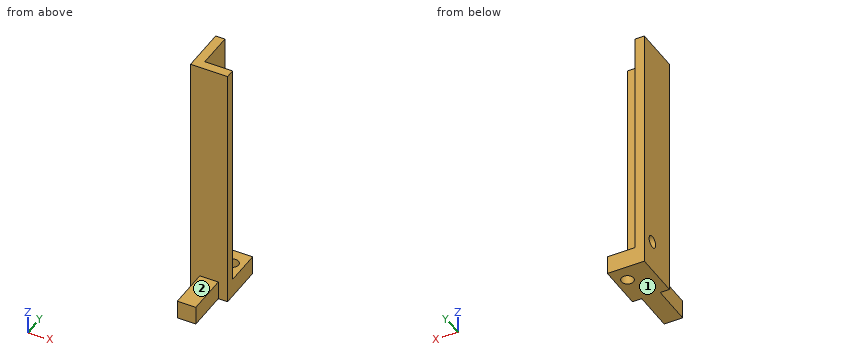
```python
from build123d import *

# Parameters (mm, degrees)
BOSS_EXTRUDE1_DEPTH      = 10
SKETCH2_W                = 30
SKETCH2_H                = 25
BOSS_EXTRUDE2_DEPTH      = 5
BOSS_EXTRUDE3_DEPTH      = 5
BOSS_EXTRUDE4_DEPTH      = 105
SKETCH7_R                = 3.25
CUT_EXTRUDE10_DEPTH      = 15
CUT_EXTRUDE10_DEPTH_BACK = 13
SKETCH8_R                = 3.25
CUT_EXTRUDE11_DEPTH      = 17
CUT_EXTRUDE11_DEPTH_BACK = 14


with BuildPart() as part:
    # Sketch1 → Boss-Extrude1 (new body)
    with BuildSketch(Plane(origin=(0, 0, 0), x_dir=(0, 0, -1), z_dir=(1, 0, 0))):
        Polygon((0, 0), (-10, 0), (-10, -20), (-30, -20), (-30, -25), (-10, -25), (-10, -47.38), (0, -47.38), align=None)
    extrude(amount=BOSS_EXTRUDE1_DEPTH)

    # Sketch2 → Boss-Extrude2 (add)
    with BuildSketch(Plane.ZY):
        with Locations((15, -12.5)):
            Rectangle(SKETCH2_W, SKETCH2_H)
    extrude(amount=BOSS_EXTRUDE2_DEPTH)

    # Sketch3 → Boss-Extrude3 (add)
    with BuildSketch(Plane(origin=(10, 0, 0), x_dir=(0, 0, -1), z_dir=(1, 0, 0))):
        Polygon((-10, 0), (-10, -20), (-30, -20), (-30, -25), (-10, -25), (0, -25), (0, 0), align=None)
    extrude(amount=BOSS_EXTRUDE3_DEPTH)

    # Sketch4 → Boss-Extrude4 (add)
    with BuildSketch(Plane.XY.offset(30)):
        Polygon((-5, 0), (-5, -25), (15, -25), (15, -20), (0, -20), (0, 0), align=None)
    extrude(amount=BOSS_EXTRUDE4_DEPTH)

    # Sketch7 → Cut-Extrude10 (cut, two sides)
    with BuildSketch(Plane(origin=(0, 0, 0), x_dir=(-1, 0, 0), z_dir=(0, 0, -1))) as cut_extrude10_sk:
        with Locations((-8.955912711, -8.964075593)):
            Circle(SKETCH7_R)
    extrude(amount=CUT_EXTRUDE10_DEPTH, mode=Mode.SUBTRACT)
    extrude(cut_extrude10_sk.sketch, amount=-CUT_EXTRUDE10_DEPTH_BACK, mode=Mode.SUBTRACT)

    # Sketch8 → Cut-Extrude11 (cut, two sides)
    with BuildSketch(Plane.ZY.offset(5)) as cut_extrude11_sk:
        with Locations((17, -8)):
            Circle(SKETCH8_R)
    extrude(amount=CUT_EXTRUDE11_DEPTH, mode=Mode.SUBTRACT)
    extrude(cut_extrude11_sk.sketch, amount=-CUT_EXTRUDE11_DEPTH_BACK, mode=Mode.SUBTRACT)


solid = part.part
```
Read the model definition and answer for the solid it produces. Units are mm, in the model's axes. Face numbers are marked on the shaded views. A direction names the side the tool comes from. Give positions to 0.01 mm unless a question says otherwise; leave off trailing zeros. Write each loop counter-clockwise with the first axis right and the second up, starting at its lowest first coordinate (ties: lowest second). Pieces come first, ordered by that corner, then holes. Notation, with made-up numbers: (37.25, -7.5) -> (81.25, -7.5) arc R24 cw to (81.25, 30.5) -> close; hole circle Ø4 at (78, -29). An arc over 180 degrees is marked (long way). Answer in a Markdown table with one row per item.
1) Section B-B on y = -17 is taken. Give the vertices of the cut face in (x, z), plus the area to 3 significant figures.
Results list:
| item | result |
|---|---|
| outline | (-5, 0) -> (15, 0) -> (15, 10) -> (0, 10) -> (0, 135) -> (-5, 135) -> close |
| area | 825 mm^2 |
2) A tool of negligible diameter and unlimited length cuts with its end or side. For the marked faces 1 and 2, from which of +Z, -Z, +X, -X, +Y, -Y can it reach the whole face along a straight path? Write none if from no direction.
Results list:
| item | result |
|---|---|
| face 1 | -Z, +X, -X, +Y, -Y |
| face 2 | +Z, +X, -X, -Y |
3) Each of these flat-tipped pins is pushed along its axis until it touches: pin 1 Ø2 at (x, z) = (0, 80) entering from -Y; pin 2 Ø3 at (x, z) = (3, 88) entering from +Y; pin 3 Ø16 at (y, z) = (-11, 57) entering from +X. Where does it stop, or does it pass through?
Results list:
| item | result |
|---|---|
| pin 1 | y = -25 |
| pin 2 | y = -20 |
| pin 3 | x = 0 |
4) Section A-A on z = 17 is taken. Give the vertices of the cut face in (x, y).
Results list:
| item | result |
|---|---|
| outline | (-5, -25) -> (15, -25) -> (15, -20) -> (0, -20) -> (0, -11.25) -> (-5, -11.25) -> close; (-5, -4.75) -> (0, -4.75) -> (0, 0) -> (-5, 0) -> close |
5) Straight lines are drawn through the part: line 1 (Y direction, x = -2.8, z = 17); line 2 (Z direction, x = 13.25, y = -8.5); line 3 (Y direction, x = -3.75, z = 109). For each, find the intervals that lie inside material, in ascending order. Write a range as [from, to].
Results list:
| item | result |
|---|---|
| line 1 | [-25, -11.25], [-4.75, 0] |
| line 2 | [0, 10] |
| line 3 | [-25, 0] |
6) Section D-D on x = 8.75 is taken. Give the vertices of the cut face in (y, z).
Results list:
| item | result |
|---|---|
| outline | (-47.38, 0) -> (-12.21, 0) -> (-12.21, 10) -> (-20, 10) -> (-20, 135) -> (-25, 135) -> (-25, 10) -> (-47.38, 10) -> close; (-5.72, 0) -> (0, 0) -> (0, 10) -> (-5.72, 10) -> close |
7) Section C-C on x = -1.5 is taken. Give the vertices of the cut face in (y, z), plus the area to 3 significant figures.
Results list:
| item | result |
|---|---|
| outline | (-25, 0) -> (0, 0) -> (0, 135) -> (-25, 135) -> close; hole circle Ø6.5 at (-8, 17) |
| area | 3,340 mm^2 |
